Autodesk Fusion 360 part; units mm, degrees
sketch "Sketch1" plane through (0, 0, 0) normal (0, 0, 1) x (1, 0, 0)
  line L0 (0, 0) -> (134, 0)
  line L1 (134, 0) -> (134, 84)
  line L2 (134, 84) -> (0, 84)
  line L3 (0, 84) -> (0, 0)
  line L4 (2, 2) -> (132, 2)
  line L5 (132, 2) -> (132, 82)
  line L6 (132, 82) -> (2, 82)
  line L7 (0, 82) -> (1.8, 82)
  line L8 (1.8, 82) -> (1.8, 73.8)
  line L9 (1.8, 73.8) -> (0, 73.8)
  line L10 (0, 73.8) -> (0, 82)
  line L11 (0, 73.8) -> (1.8, 73.8)
  line L12 (1.8, 73.8) -> (1.8, 10.2)
  line L13 (1.8, 10.2) -> (0, 10.2)
  line L14 (0, 10.2) -> (0, 73.8)
  line L15 (4.4, 73.8) -> (4.4, 72.6661)
  line L16 (2, 72.6661) -> (2, 73.8)
  line L17 (4.4, 73.8) -> (6.2, 73.8)
  line L18 (6.2, 73.8) -> (6.2, 10.2)
  line L19 (6.2, 10.2) -> (4.4, 10.2)
  line L20 (4.4, 10.2) -> (4.4, 73.8)
  line L21 (2, 82) -> (1.8, 82)
  line L22 (1.8, 10.2) -> (1.8, 2)
  line L23 (2, 2) -> (1.8, 2)
  line L24 (1.8, 2) -> (12.8, 2)
  line L25 (12.8, 2) -> (15.8, 2)
  line L26 (15.8, 2) -> (15.8, 3)
  line L27 (15.8, 3) -> (12.8, 3)
  line L28 (12.8, 3) -> (12.8, 2)
  line L29 (12.8, 82) -> (15.8, 82)
  line L30 (15.8, 82) -> (15.8, 81)
  line L31 (15.8, 81) -> (12.8, 81)
  line L32 (12.8, 81) -> (12.8, 82)
  line L33 (132, 82) -> (121, 82)
  line L34 (132, 82) -> (132, 71)
  line L35 (121, 82) -> (118, 82)
  line L36 (118, 82) -> (118, 81)
  line L37 (118, 81) -> (121, 81)
  line L38 (121, 81) -> (121, 82)
  line L39 (132, 71) -> (131, 71)
  line L40 (131, 71) -> (131, 68)
  line L41 (131, 68) -> (132, 68)
  line L42 (132, 68) -> (132, 71)
  line L43 (132, 2) -> (132, 13)
  line L44 (132, 2) -> (121, 2)
  line L45 (132, 13) -> (131, 13)
  line L46 (131, 13) -> (131, 16)
  line L47 (131, 16) -> (132, 16)
  line L48 (132, 16) -> (132, 13)
  line L49 (121, 2) -> (118, 2)
  line L50 (118, 2) -> (118, 3)
  line L51 (118, 3) -> (121, 3)
  line L52 (121, 3) -> (121, 2)
  dimension "d1" = 134
  dimension "d2" = 84
  dimension "d33" = 130
  dimension "d34" = 80
  dimension "d35" = 1.8
  dimension "d36" = 8.2
  dimension "d37" = 63.6
  dimension "d38" = 2.4
  dimension "d39" = 1.8
  dimension "d41" = 11
  dimension "d42" = 3
  dimension "d43" = 1
  dimension "d44" = 1
  dimension "d45" = 11
  dimension "d46" = 11
  dimension "d47" = 3
  dimension "d48" = 11
  dimension "d49" = 11
  dimension "d50" = 1
  dimension "d51" = 3
extrude "Extrude1" add sketch "Sketch1" along normal blind 2 contours L0 L1 L2 L3 L4 L5 L6 L7 L13 L21 L22 L23 L24 L25 L29 L33 L34 L35 L42 L43 L44 L48 L49 | L3 L9 L11 L12 L13 L14 | L3 L7 L8 L9 L10 L11 | L4 L5 L6 L8 L12 L21 L22 L23 L24 L26 L27 L28 L30 L31 L32 L33 L34 L36 L37 L38 L39 L40 L41 L43 L44 L45 L46 L47 L50 L51 L52 | L4 L25 L26 L27 L28 | L6 L29 L30 L31 L32 | L4 L49 L50 L51 L52 | L6 L35 L36 L37 L38 | L5 L45 L46 L47 L48 | L5 L39 L40 L41 L42 | L15 L17 L18 L19 L20
extrude "Extrude7" add sketch "Sketch1" along normal blind 5 contours L4 L25 L26 L27 L28 | L6 L29 L30 L31 L32 | L4 L49 L50 L51 L52 | L6 L35 L36 L37 L38 | L5 L45 L46 L47 L48 | L5 L39 L40 L41 L42
extrude "Extrude8" add sketch "Sketch1" along normal blind 4 contours L3 L9 L11 L12 L13 L14 | L15 L17 L18 L19 L20
sketch "Sketch8" plane through (0, 2, 0) normal (0, -1, 0) x (1, 0, 0)
  line L0 (12.8, 2) -> (15.8, 2)
  line L1 (15.8, 2) -> (15.8, 5)
  line L2 (15.8, 5) -> (12.8, 5)
  line L3 (12.8, 5) -> (12.8, 2)
  line L4 (12.8, 5) -> (15.8, 5)
  line L5 (15.8, 5) -> (15.8, 4)
  line L6 (15.8, 4) -> (12.8, 4)
  line L7 (12.8, 4) -> (12.8, 5)
  line L8 (118.0033, 5) -> (121.0033, 5)
  line L9 (121.0033, 5) -> (121.0033, 4)
  line L10 (121.0033, 4) -> (118.0033, 4)
  line L11 (118.0033, 4) -> (118.0033, 5)
  dimension "d56" = 1
  dimension "d57" = 3
  dimension "d58" = 1
extrude "Extrude9" add sketch "Sketch8" along normal blind 1 contours L1 L2 L3 L4 L5 L6 L7 | L8 L9 L10 L11
sketch "Sketch9" plane through (132, 0, 0) normal (1, 0, 0) x (0, 1, 0)
  line L0 (13, 2) -> (16, 2)
  line L1 (16, 2) -> (16, 5)
  line L2 (16, 5) -> (13, 5)
  line L3 (13, 5) -> (13, 2)
  line L4 (13, 5) -> (16, 5)
  line L5 (16, 5) -> (16, 4)
  line L6 (16, 4) -> (13, 4)
  line L7 (13, 4) -> (13, 5)
  line L8 (68, 5) -> (71, 5)
  line L9 (71, 5) -> (71, 4)
  line L10 (71, 4) -> (68, 4)
  line L11 (68, 4) -> (68, 5)
  dimension "d61" = 3
  dimension "d62" = 1
  dimension "d63" = 3
  dimension "d64" = 1
extrude "Extrude10" add sketch "Sketch9" along normal blind 1 contours L1 L2 L3 L4 L5 L6 L7 | L8 L9 L10 L11
sketch "Sketch10" plane through (0, 82, 0) normal (0, 1, 0) x (-1, 0, 0)
  line L0 (-121, 2) -> (-118, 2)
  line L1 (-118, 2) -> (-118, 5)
  line L2 (-118, 5) -> (-121, 5)
  line L3 (-121, 5) -> (-121, 2)
  line L4 (-15.8, 5) -> (-12.8, 5)
  line L5 (-12.8, 5) -> (-12.8, 4)
  line L6 (-12.8, 4) -> (-15.8, 4)
  line L7 (-15.8, 4) -> (-15.8, 5)
  line L8 (-121, 5) -> (-118, 5)
  line L9 (-118, 5) -> (-118, 4)
  line L10 (-118, 4) -> (-121, 4)
  line L11 (-121, 4) -> (-121, 5)
  dimension "d67" = 3
  dimension "d68" = 1
  dimension "d69" = 3
  dimension "d70" = 1
extrude "Extrude11" add sketch "Sketch10" along normal blind 1 contours L1 L2 L3 L8 L9 L10 L11 | L4 L5 L6 L7
fillet "Fillet2" radius 0.5 12 edges at (119.5, 83, 5) (119.5, 83, 4) (133, 69.5, 5) (133, 69.5, 4) (133, 14.5, 5) (133, 14.5, 4) (119.5033, 1, 5) (14.3, 83, 5) (14.3, 83, 4) (14.3, 1, 5) (14.3, 1, 4) (119.5033, 1, 4)
equation "d35 = 2 mm - 0.2 mm"
equation "d37 = 80 mm - ( 8.2 * 2 ) * 1 mm"
equation "d41 = 15 mm - 3 mm - 1 mm"
equation "d52 = 3 mm + 2 mm"
equation "d54 = 2 mm + 2 mm"
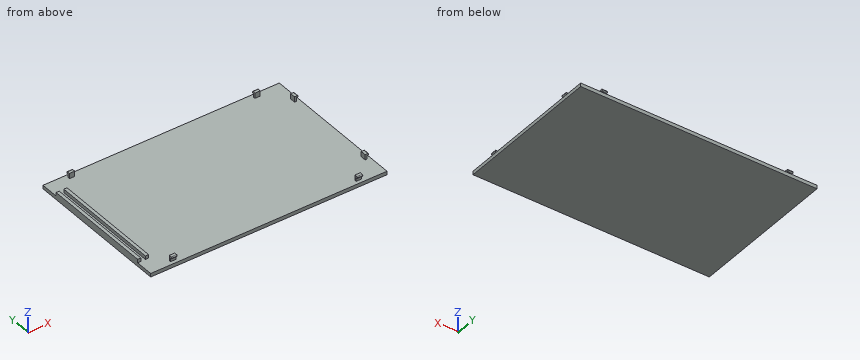
Could you check a few things on this model? Use its own coordinates, in mm. Round coordinates to 2 decimals unless told otherwise and drop trailing zeros. Write each loop counter-clockwise with the first axis right and the second up, starting at its lowest first coordinate (ties: lowest second). Pieces come first, ordered by that corner, then holes. Notation, with made-up numbers: (41, 22.5) -> (98, 22.5) arc R21 cw to (98, 58.5) -> close; hole circle Ø2 at (46, 59). An arc over 180 degrees is marked (long way). Use a Markdown table: item, result.
1. If we section it at B-B (x = 115): List the corners of the cut face in (y, z) for me.
Answer key:
| item | result |
|---|---|
| outline | (0, 0) -> (84, 0) -> (84, 2) -> (0, 2) -> close |
2. For pin 1 Ø0.5 at (x, z) = (5.5, 3.5) entering from -Y; pin 2 Ø10 at (x, y) = (75.5, 25.5) entering from +Z; pin 3 Ø0.6 at (y, z) = (70, 2.5) entering from +X, each with a flat end and sliding along its axis, tell me the tip position at first contact or that it passes through.
Answer key:
| item | result |
|---|---|
| pin 1 | stops at y = 10.2 |
| pin 2 | stops at z = 2 |
| pin 3 | stops at x = 132 |
3. Please list where these lines run through material, in increasing order: probe 1 along X at (y, z) = (37, 2.7); probe 2 along Z at (x, y) = (110.5, 76.5).
Answer key:
| item | result |
|---|---|
| probe 1 | x = 0 to 1.8, 4.4 to 6.2 |
| probe 2 | z = 0 to 2 |
4. If we section it at A-A (y = 36): List the corners of the cut face in (x, z) for me, then the cut area to 3 significant figures.
Answer key:
| item | result |
|---|---|
| outline | (0, 0) -> (134, 0) -> (134, 2) -> (6.2, 2) -> (6.2, 4) -> (4.4, 4) -> (4.4, 2) -> (1.8, 2) -> (1.8, 4) -> (0, 4) -> close |
| area | 275 mm^2 |
5. If we section it at C-C (y = 78): List the corners of the cut face in (x, z) for me.
Answer key:
| item | result |
|---|---|
| outline | (0, 0) -> (134, 0) -> (134, 2) -> (0, 2) -> close |
